Autodesk Fusion 360 part; units mm, degrees
sketch "Sketch1" plane through (0, 0, 0) normal (0, 1, 0) x (1, 0, 0)
  line L0 (7.5, -3.5) -> (0, -3.5)
  line L1 (3.5, 3.5) -> (7.5, 3.5)
  line L2 (7.5, 3.5) -> (12.5, 2.5)
  line L3 (7.5, -3.5) -> (12.5, -2.5)
  line L4 (12.5, 2.5) -> (22, 2.5)
  line L5 (12.5, -2.5) -> (22, -2.5)
  line L6 (22.5, 2) -> (22.5, -2)
  line L7 (57.5, -1) -> (22.5, -1)
  line L8 (22.5, 1) -> (57.5, 1)
  line L9 (57.5, 1) -> (57.5, -1)
  line L10 (70.5, -2) -> (58.5, -2)
  line L11 (58.5, 2) -> (70.5, 2)
  line L12 (72.5, 0) -> (72.5, 0) construction
  line L13 (57.5, 1) -> (57.5, 1) construction
  line L14 (57.5, -1) -> (57.5, -1) construction
  arc A0 (58.5, 2) -> (57.5, 1) centre (58.5, 1) ccw
  arc A1 (57.5, -1) -> (58.5, -2) centre (58.5, -1) ccw
  arc A2 (72.5, 0) -> (70.5, 2) centre (70.5, 0) ccw
  arc A3 (70.5, -2) -> (72.5, 0) centre (70.5, 0) ccw
  line L15 (1.5764, 12.5) -> (0, 12.5)
  line L16 (3.5, 3.5) -> (2.0696, 12.0822)
  arc A4 (22.5, 2) -> (22, 2.5) centre (22, 2) ccw
  arc A5 (22, -2.5) -> (22.5, -2) centre (22, -2) ccw
  line L17 (-7.5, -3.5) -> (-12.5, -2.5)
  line L18 (-12.5, -2.5) -> (-22, -2.5)
  arc A6 (-22.5, -2) -> (-22, -2.5) centre (-22, -2) ccw
  line L19 (-22.5, 2) -> (-22.5, -2)
  arc A7 (-22, 2.5) -> (-22.5, 2) centre (-22, 2) ccw
  line L20 (-12.5, 2.5) -> (-22, 2.5)
  line L21 (-7.5, 3.5) -> (-12.5, 2.5)
  line L22 (-3.5, 3.5) -> (-7.5, 3.5)
  line L23 (-1.5764, 12.5) -> (0, 12.5)
  line L24 (-3.5, 3.5) -> (-2.0696, 12.0822)
  line L25 (-7.5, -3.5) -> (0, -3.5)
  line L26 (-22.5, 1) -> (-57.5, 1)
  line L27 (-57.5, -1) -> (-22.5, -1)
  arc A8 (-57.5, 1) -> (-58.5, 2) centre (-58.5, 1) ccw
  arc A9 (-70.5, 2) -> (-72.5, 0) centre (-70.5, 0) ccw
  arc A10 (-72.5, 0) -> (-70.5, -2) centre (-70.5, 0) ccw
  line L28 (-70.5, -2) -> (-58.5, -2)
  arc A11 (-58.5, -2) -> (-57.5, -1) centre (-58.5, -1) ccw
  line L29 (-58.5, 2) -> (-70.5, 2)
  line L30 (-57.5, 1) -> (-57.5, -1)
  arc A12 (-1.5764, 12.5) -> (-2.0696, 12.0822) centre (-1.5764, 12) ccw
  arc A13 (2.0696, 12.0822) -> (1.5764, 12.5) centre (1.5764, 12) ccw
  line L31 (-3.5, 3.5) -> (3.5, 3.5)
  line L32 (-72.5, 0) -> (72.5, 0)
  line L33 (0, 12.5) -> (0, 3.5)
  point P0 (0, 3.5)
  dimension "d28" = 7
  dimension "d37" = 1
  dimension "d38" = 1
  dimension "d39" = 2
  dimension "d40" = 2
  dimension "d43" = 0.5
  dimension "d44" = 0.5
  dimension "d45" = 0.5
  dimension "d46" = 0.5
revolve "Revolve2" add sketch "Sketch1" angle 360 about axis through (0, 0, -12.5) along (0, 0, 1) contours L15 L16 A13 L31 L33 makes body 1
revolve "Revolve1" add sketch "Sketch1" angle 360 about axis through (-72.5, 0, 0) along (1, 0, 0) separate body contours L1 L2 L4 L6 A4 L19 A7 L20 L21 L22 L31 L32 | L6 L8 L9 L32 | L19 L26 L30 L32 | L9 L11 A0 A2 L32 | A8 A9 L29 L30 L32 makes body 2
extrude "Extrude1" add 1 faces at (-0.8429, -2.1478, -3.5) along direction (0, 0, 1) blind 3.5 on bodies 1 bodies 1 2
Source: CAD feature listing. Evaluate the final solid. Frame: model axes, mm. A direction names the side the tool comes from. Give positions to 0.01 mm unless a question says otherwise; leave off trailing zeros. Write each loop counter-clockwise with the first axis right and the second up, starting at its lowest first coordinate (ties: lowest second). Pieces come first, ordered by that corner, then holes. Notation, with made-up numbers: (44, 27) - (101, 27) arc R21 cw to (101, 36) - close; hole circle Ø8 at (31.5, 48). An arc over 180 degrees is marked (long way). One line per item, written item: value. Start each with the question number.
Q1. Section query A-A, the plane x = 0. Return the cut outline in (y, z), then the cut area to 3 significant figures.
Q2. First-contact query: pin 1 Ø5 at (x, z) = (18.5, -0.5) entering from +Y; pin 2 Ø3 at (x, y) = (14.5, 0) entering from -Z; pin 3 Ø1.5 at (y, z) = (-2, 1) entering from +X. Flat tips, straight axial feed; report the tip coordinate or a pass-through.
Q3. Material intervals for probe 1 along X at (y, z) = (-2, -11); probe 2 along Y at (x, z) = (-14.5, 0); probe 3 along Z at (x, y) = (5.5, -3), sorted ascending. Write a range as from..to.
Q4. Set-up query: faces 1 (the face through (-17.32, 2.44, 0.54)), 2 (the face through (22.5, -1, -1)), 3 (the face through (0, 3.5, -2.5)). Return all of +Z, -Z, +X, -X, +Y, -Y with unobstructed straight access to the full face (end or side cutting, diameter ignored); none if empty.
Q5. Section query C-C, the plane x = 42.5. Return the cut outline in (y, z), then the cut area to 3 significant figures.
Q6. Section query B-B, the plane z = -5.75. Return the cut outline in (x, y) (3 decimals).
Answer:
1. outline: (-3.5, -3.5) - (-2.07, -12.08) arc R0.5 ccw to (-1.58, -12.5) - (1.58, -12.5) arc R0.5 ccw to (2.07, -12.08) - (3.5, -3.5) - (3.5, 0) arc R3.5 ccw to (-3.5, 0) - close
1. area: 93.2 mm2
2. pin 1: stops at y = 2.5
2. pin 2: stops at z = -2.5
2. pin 3: stops at x = 71.84
3. probe 1: x = -1.03..1.03
3. probe 2: y = -2.5..2.5
3. probe 3: z = -1.8..1.8
4. face 1: -X
4. face 2: none
4. face 3: -Z, +Y
5. outline: circle Ø2 at (0, 0)
5. area: 3.14 mm2
6. outline: circle Ø6.25 at (0, 0)
